```python
from build123d import *

# Parameters (mm, degrees)
SKETCH1_R           = 2.413
BOSS_EXTRUDE1_DEPTH = 2.54
SKETCH2_R           = 3.175
CUT_EXTRUDE1_DEPTH  = 3.54


with BuildPart() as part:
    # Sketch1 → Boss-Extrude1 (new body)
    with BuildSketch(Plane(origin=(0, 0, 0), x_dir=(1, 0, 0), z_dir=(0, 1, 0))):
        Polygon((-74.6125, -11.1125), (-74.6125, 11.1125), (-42.8625, 11.1125), (-11.1125, 42.8625), (-11.1125, 74.6125), (11.1125, 74.6125), (11.1125, 42.8625), (42.8625, 11.1125), (74.6125, 11.1125), (74.6125, -11.1125), (42.8625, -11.1125), (11.1125, -42.8625), (11.1125, -74.6125), (-11.1125, -74.6125), (-11.1125, -42.8625), (-42.8625, -11.1125), align=None)
        with Locations((-23.8125, 2.778125)):
            Circle(SKETCH1_R, mode=Mode.SUBTRACT)
        with Locations((-63.1825, -2.778125)):
            Circle(SKETCH1_R, mode=Mode.SUBTRACT)
        with Locations((-2.778125, 63.1825)):
            Circle(SKETCH1_R, mode=Mode.SUBTRACT)
        with Locations((2.778125, 23.8125)):
            Circle(SKETCH1_R, mode=Mode.SUBTRACT)
        with Locations((63.1825, 2.778125)):
            Circle(SKETCH1_R, mode=Mode.SUBTRACT)
        with Locations((23.8125, -2.778125)):
            Circle(SKETCH1_R, mode=Mode.SUBTRACT)
        with Locations((2.778125, -63.1825)):
            Circle(SKETCH1_R, mode=Mode.SUBTRACT)
        with Locations((-2.778125, -23.8125)):
            Circle(SKETCH1_R, mode=Mode.SUBTRACT)
    extrude(amount=BOSS_EXTRUDE1_DEPTH)

    # Sketch2 → Cut-Extrude1 (cut, through all)
    with BuildSketch(Plane(origin=(0, 2.54, 0), x_dir=(1, 0, 0), z_dir=(0, 1, 0))):
        Circle(SKETCH2_R)
    extrude(amount=-CUT_EXTRUDE1_DEPTH, mode=Mode.SUBTRACT)


solid = part.part
```
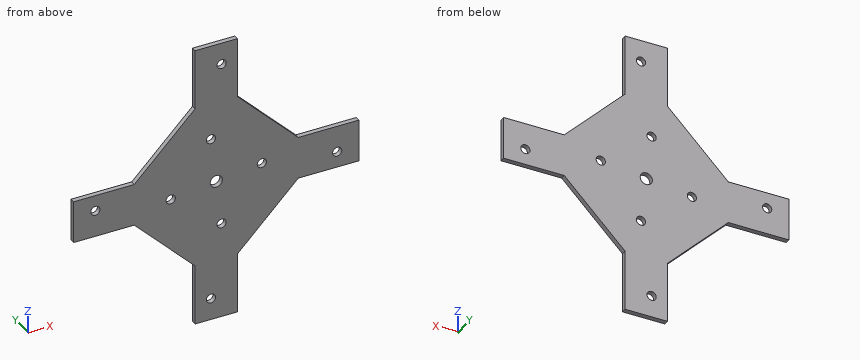
The listing builds one solid part. Answer for the finished solid, in the listing's coordinates (mm). Coordinates: 2 decimals unless noted, no trailing zeros. Loops run counter-clockwise (first coordinate to the right, second up) from the corner with the lowest first, then second, coordinate; pieces in that order, holes last. Notation, with made-up numbers: M 39.5,70.5 L 77.5,70.5 A5 ccw 77.5,77.5 Z; hole C 48,53 d8. An arc over 180 degrees is marked long. Answer as a JSON object with one key per item and string values. Group by question number.
Item 1: Each of these flat-tipped pins is pushed along its axis until it touches: P1, Ø0.8, axis at x = 60, y = 1.5, coming from the -Z side; P2, Ø1.3, axis at x = -61, y = 1, coming from the +Z side; P3, Ø0.8, axis at y = 1, z = -60.5, coming from the -X side. Where does it stop, or does it pass through?
Item 2: Section B-B (x = -53) is taken. Write down the section's boundary in (y, z), and give its area (3 significant figures).
Item 3: Consider L1, parallel to Z at x = 0, y = 1 (1 decimal); L2, parallel to Z at x = -3.5, y = 1.9 (1 decimal); L3, parallel to X at y = 1.5, z = 4.5. Determine where each line is inside the solid, lowest interval first.
Item 4: Section A-A (y = 0.8) is taken. Give the number of separate pieces and of enclosed holes in the cut face, and give its area (3 significant figures).
Item 5: Section C-C (z = 45) is taken. Write down the section's boundary in (x, y).
Solved:
{
 "1": {"P1": "stops at z = -11.11", "P2": "stops at z = 11.11", "P3": "stops at x = -11.11"},
 "2": {"outline": "M 0,-11.11 L 2.54,-11.11 L 2.54,11.11 L 0,11.11 Z", "area": "56.5 mm2"},
 "3": {"L1": "z = -74.6 to -3.2, 3.2 to 74.6", "L2": "z = -74.6 to -65.5, -60.9 to 21.5, 26.1 to 74.6", "L3": "x = -74.61 to -64.87, -61.49 to 22.12, 25.5 to 74.61"},
 "4": {"separate pieces": "1", "enclosed holes": "9", "area": "7,980 mm2"},
 "5": {"outline": "M -11.11,0 L 11.11,0 L 11.11,2.54 L -11.11,2.54 Z"}
}
